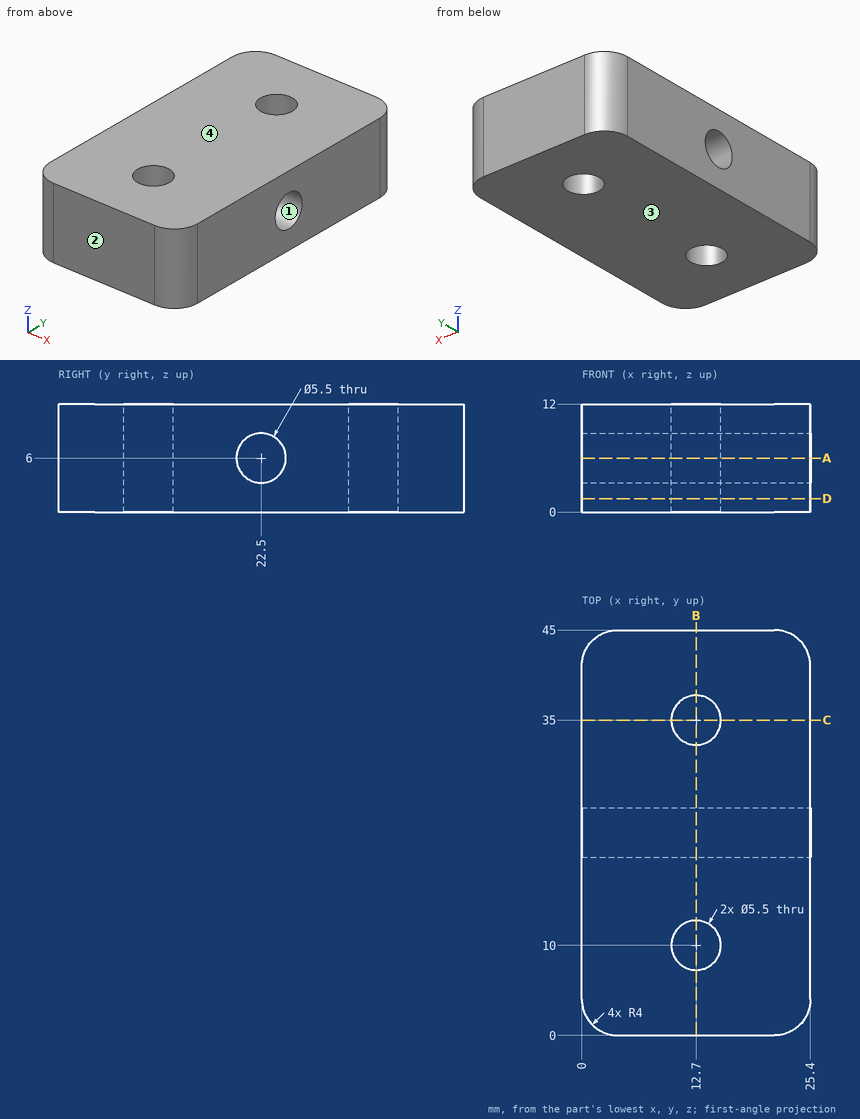
For this review, use the dimensioned drawing (mm, ordinates from the lowest corner) and the shaded views. Give positions to 0.01 mm unless a question says otherwise; leave off trailing zeros. Order: outer loops, then holes, each group sorted by start corner. A loop starts at its lowest first (then second) coordinate and runs counter-clockwise, first axis right, second up. Notation, with made-up numbers: (-1, 46) - (38, 46) arc R21 ccw to (38, 83) - close; hole circle Ø1 at (8.5, -5.75). An arc over 180 degrees is marked (long way). Write item = value, one per line. Start each with the question number.
Q1. We need section B-B on x = 12.7. State the section outline as (y, z) points.
Q2. We need section A-A on z = 6. State the section outline as (x, y) points, plus the area to 3 significant figures.
Q3. Clearance check with a flat-ended pin moving along its axis: pin 1 Ø3.5 at (x, y) = (12.7, 35) entering from -Z. State where the tip first meets the part, or that it passes through.
Q4. We need section C-C on y = 35. State the section outline as (x, z) points.
Q5. We need section D-D on z = 1.5. State the section outline as (x, y) points.
Q6. Mouldability with a two-part tool opening along Z and no side actions: class the marked faces 1, 2, 3 and 4 as released by +Z, released by -Z, zero draft, split by the parting line, or undercut.
Q7. To check wall thickness, follow L1, parallel to Y at x = 12.7, z = 9.25; L2, parallel to Y at x = 12.7, z = 6; L3, parallel to Y at x = 8, z = 6. State the ranges of each line that lie inside material, in increasing order. Write a range as from..to.
Working result:
q1.outline = (0, 0) - (7.25, 0) - (7.25, 12) - (0, 12) - close; (12.75, 0) - (32.25, 0) - (32.25, 12) - (12.75, 12) - close; (37.75, 0) - (45, 0) - (45, 12) - (37.75, 12) - close; hole circle Ø5.5 at (22.5, 6)
q2.outline = (0, 4) arc R4 ccw to (4, 0) - (21.4, 0) arc R4 ccw to (25.4, 4) - (25.4, 19.75) - (0, 19.75) - close; (0, 25.25) - (25.4, 25.25) - (25.4, 41) arc R4 ccw to (21.4, 45) - (4, 45) arc R4 ccw to (0, 41) - close; hole circle Ø5.5 at (12.7, 10); hole circle Ø5.5 at (12.7, 35)
q2.area = 942 mm²
q3.pin_1 = through
q4.outline = (0, 0) - (9.95, 0) - (9.95, 12) - (0, 12) - close; (15.45, 0) - (25.4, 0) - (25.4, 12) - (15.45, 12) - close
q5.outline = (0, 4) arc R4 ccw to (4, 0) - (21.4, 0) arc R4 ccw to (25.4, 4) - (25.4, 41) arc R4 ccw to (21.4, 45) - (4, 45) arc R4 ccw to (0, 41) - close; hole circle Ø5.5 at (12.7, 10); hole circle Ø5.5 at (12.7, 35)
q6.face_1 = undercut
q6.face_2 = zero draft
q6.face_3 = released by -Z
q6.face_4 = released by +Z
q7.L1 = 0..7.25, 12.75..32.25, 37.75..45
q7.L2 = 0..7.25, 12.75..19.75, 25.25..32.25, 37.75..45
q7.L3 = 0..19.75, 25.25..45
